```python
from build123d import *

# Parameters (mm, degrees)
F0_W          = 43
F0_H          = 43
F0_R          = 1.75
F0_R_2        = 16
F1_DEPTH      = 4
F2_R          = 5
F3_SIZE       = 3
F4_DEPTH      = 4
F4_DEPTH_BACK = 2


with BuildPart() as f1:
    # F0 (on Top) → F1 (new body)
    with BuildSketch(Plane.XY):
        Polygon((-8.6166327415, 27.9440277213), (-55.6166327415, 27.9440277213), (-55.6166327415, -32.0559722787), (58.3833672585, -32.0559722787), (58.3833672585, 27.9440277213), (11.3833672585, 27.9440277213), (11.3833672585, 43.9440277213), (-8.6166327415, 43.9440277213), align=None)
        with Locations((-30.6166327415, -4.2559722787)):
            Rectangle(F0_W, F0_H, mode=Mode.SUBTRACT)
        with Locations((29.9833672585, -4.2559722787)):
            Rectangle(F0_W, F0_H, mode=Mode.SUBTRACT)
        with BuildLine():
            ThreePointArc((-0.6166327415, 29.9440277213), (1.3833672585, 31.9440277213), (3.3833672585, 29.9440277213))
            Line((3.3833672585, 29.9440277213), (3.3833672585, 24.9440277213))
            ThreePointArc((3.3833672585, 24.9440277213), (1.3833672585, 22.9440277213), (-0.6166327415, 24.9440277213))
            Line((-0.6166327415, 24.9440277213), (-0.6166327415, 29.9440277213))
        make_face(mode=Mode.SUBTRACT)
        with Locations((-30.6166327415, -4.2559722787)):
            Rectangle(F0_W, F0_H)
        with Locations((-46.1166327415, -19.7559722787)):
            Circle(F0_R, mode=Mode.SUBTRACT)
        with Locations((-15.1166327415, -19.7559722787)):
            Circle(F0_R, mode=Mode.SUBTRACT)
        with Locations((-30.6166327415, -4.2559722787)):
            Circle(F0_R_2, mode=Mode.SUBTRACT)
        with Locations((-46.1166327415, 11.2440277213)):
            Circle(F0_R, mode=Mode.SUBTRACT)
        with Locations((-15.1166327415, 11.2440277213)):
            Circle(F0_R, mode=Mode.SUBTRACT)
        with Locations((29.9833672585, -4.2559722787)):
            Rectangle(F0_W, F0_H)
        with Locations((14.4833672585, -19.7559722787)):
            Circle(F0_R, mode=Mode.SUBTRACT)
        with Locations((45.4833672585, -19.7559722787)):
            Circle(F0_R, mode=Mode.SUBTRACT)
        with Locations((29.9833672585, -4.2559722787)):
            Circle(F0_R_2, mode=Mode.SUBTRACT)
        with Locations((14.4833672585, 11.2440277213)):
            Circle(F0_R, mode=Mode.SUBTRACT)
        with Locations((45.4833672585, 11.2440277213)):
            Circle(F0_R, mode=Mode.SUBTRACT)
    extrude(amount=F1_DEPTH)

    # F2
    f2_edges = [f1.edges().sort_by_distance(p)[0] for p in [
        (-8.616633, 43.944028, 2),
        (-8.616633, 27.944028, 2),
        (-55.616633, 27.944028, 2),
        (11.383367, 43.944028, 2),
        (11.383367, 27.944028, 2),
        (58.383367, 27.944028, 2),
    ]]
    fillet(f2_edges, radius=F2_R)

    # F3
    f3_edges = [f1.edges().sort_by_distance(p)[0] for p in [
        (1.383367, -32.055972, 4),
    ]]
    chamfer(f3_edges, length=F3_SIZE)

    # F0 (on Top) → F4 (cut, two sides)
    with BuildSketch(Plane.XY) as f4_sk:
        with Locations((-30.6166327415, -4.2559722787)):
            Rectangle(F0_W, F0_H)
        with Locations((-46.1166327415, -19.7559722787)):
            Circle(F0_R, mode=Mode.SUBTRACT)
        with Locations((-15.1166327415, -19.7559722787)):
            Circle(F0_R, mode=Mode.SUBTRACT)
        with Locations((-30.6166327415, -4.2559722787)):
            Circle(F0_R_2, mode=Mode.SUBTRACT)
        with Locations((-46.1166327415, 11.2440277213)):
            Circle(F0_R, mode=Mode.SUBTRACT)
        with Locations((-15.1166327415, 11.2440277213)):
            Circle(F0_R, mode=Mode.SUBTRACT)
        with Locations((29.9833672585, -4.2559722787)):
            Rectangle(F0_W, F0_H)
        with Locations((14.4833672585, -19.7559722787)):
            Circle(F0_R, mode=Mode.SUBTRACT)
        with Locations((45.4833672585, -19.7559722787)):
            Circle(F0_R, mode=Mode.SUBTRACT)
        with Locations((29.9833672585, -4.2559722787)):
            Circle(F0_R_2, mode=Mode.SUBTRACT)
        with Locations((14.4833672585, 11.2440277213)):
            Circle(F0_R, mode=Mode.SUBTRACT)
        with Locations((45.4833672585, 11.2440277213)):
            Circle(F0_R, mode=Mode.SUBTRACT)
    extrude(amount=-F4_DEPTH, mode=Mode.SUBTRACT)
    extrude(f4_sk.sketch, amount=F4_DEPTH_BACK, mode=Mode.SUBTRACT)


solid = f1.part
```
Geometry check sheet. Reference: the model listing, model coordinates, mm. A direction names the side the tool comes from. Coordinates: 2 decimals unless noted, no trailing zeros. Loops run counter-clockwise (first coordinate to the right, second up) from the corner with the lowest first, then second, coordinate; pieces in that order, holes last. Notation, with made-up numbers: (-8, -31) - (24, -31) arc R18 ccw to (24, -7) - close; hole circle Ø11 at (-21, 74.5). An arc over 180 degrees is marked (long way). One line per item, written item: value. Start each with the question number.
(1) Mould release check, pull along Y, two halves, no side actions. Record for faces 1 (the flat face through (-8.617, 36, 2)), 2 (the cylindrical face through (-54.11, 26.52, 2.03)), 3 (the cylindrical face through (-47.865, -19.679, 2.986)): released by +Y, released by -Y, zero draft, split by the parting line, or undercut.
(2) Cross-section at D-D on x = -31. Enter the section's corners in (y, z), plus the area to 3 significant figures.
(3) Cross-section at C-C on y = -13. Enter the section's corners in (x, z), plus the area to 3 significant figures.
(4) Cross-section at A-A on x = 35. Enter the section's corners in (y, z), plus the area to 3 significant figures.
(5) Cross-section at B-B on y = 7. Enter the section's corners in (x, z), plus the area to 3 significant figures.
(6) Depth check by flat-ended pin: P1, Ø1, axis at x = 20, z = 1, coming from the +Y side; P2, Ø2, axis at y = 35.5, z = 2.5, coming from the -X side; P3, Ø8, axis at x = -17, y = -5, coming from the -Z side. Enter the tip coordinate at first touch or a pass-through.
(7) Material ranges on line 1 (X direction, y = 14, z = 1.5); line 2 (X direction, y = -11.5, z = 3.05); line 3 (Y direction, x = 13, z = 2.9), recorded low to high. Write a range as [from, to].
(8) Tool access check on faces 4 (the cylindrical face through (1.427, 22.945, 1.972)), 5 (the flat face through (39, -18, 2)), 6 (the flat face through (-32, 27.944, 2)), 7 (the flat face through (1, 43.944, 2)). Record the directions out of +Z, -Z, +X, -X, +Y, -Y that give a thin tool (end or side, any length) a straight path to the whole face; none if there is none.
Results below:
1. face 1: zero draft
1. face 2: released by +Y
1. face 3: undercut
2. outline: (-32.06, 0) - (-25.76, 0) - (-25.76, 2) - (-20.25, 2) - (-20.25, 4) - (-29.06, 4) - (-32.06, 1) - close; (11.74, 2) - (17.24, 2) - (17.24, 0) - (27.94, 0) - (27.94, 4) - (11.74, 4) - close
2. area: 85.5 mm2
3. outline: (-55.62, 0) - (-52.12, 0) - (-52.12, 2) - (-44.02, 2) - (-44.02, 4) - (-55.62, 4) - close; (-17.22, 2) - (-9.12, 2) - (-9.12, 0) - (8.48, 0) - (8.48, 2) - (16.58, 2) - (16.58, 4) - (-17.22, 4) - close; (43.38, 2) - (51.48, 2) - (51.48, 0) - (58.38, 0) - (58.38, 4) - (43.38, 4) - close
3. area: 177 mm2
4. outline: (-32.06, 0) - (-25.76, 0) - (-25.76, 2) - (-19.45, 2) - (-19.45, 4) - (-29.06, 4) - (-32.06, 1) - close; (10.94, 2) - (17.24, 2) - (17.24, 0) - (27.94, 0) - (27.94, 4) - (10.94, 4) - close
4. area: 88.7 mm2
5. outline: (-55.62, 0) - (-52.12, 0) - (-52.12, 2) - (-41.99, 2) - (-41.99, 4) - (-55.62, 4) - close; (-19.25, 2) - (-9.12, 2) - (-9.12, 0) - (8.48, 0) - (8.48, 2) - (18.61, 2) - (18.61, 4) - (-19.25, 4) - close; (41.35, 2) - (51.48, 2) - (51.48, 0) - (58.38, 0) - (58.38, 4) - (41.35, 4) - close
5. area: 193 mm2
6. P1: stops at y = 27.94
6. P2: stops at x = -8.62
6. P3: stops at z = 2
7. line 1: x = [-55.62, -52.12], [-9.12, 8.48], [51.48, 58.38]
7. line 2: x = [-55.62, -44.88], [-16.35, 15.72], [44.25, 58.38]
7. line 3: y = [-30.16, -20.68], [-18.83, 10.32], [12.17, 29.26]
8. face 4: +Z, -Z
8. face 5: -Z
8. face 6: +Z, -Z, -X, +Y
8. face 7: +Z, -Z, +X, -X, +Y
